Geometry check sheet. Reference: the model listing, model coordinates, mm. A direction names the side the tool comes from. Round coordinates to 2 decimals unless told otherwise and drop trailing zeros. Write each loop counter-clockwise with the first axis right and the second up, starting at its lowest first coordinate (ties: lowest second). Pieces come first, ordered by that corner, then holes.
Item 1: Cross-section at C-C (y = 29). Enter the section's corners in (x, z).
Item 2: Depth check by flat-ended pin: P1, Ø8, axis at x = 99, z = 47.5, coming from the +Y side; P2, Ø3, axis at x = 0.5, y = 48.5, coming from the +Z side; P3, Ø1.2, axis at x = 0.5, z = 57, coming from the +Y side. Enter the tip coordinate at first touch or a pass-through.
Item 3: Cross-section at A-A (x = -17.5). Enter the section's corners in (y, z), then the cut area to 3 significant figures.
Item 4: Access from +Z, -Z, +X, -X, +Y, -Y to the whole of each face (thin tool, end or side, straight path). Record for faces 1 (the face through (-83.213, 5.43, 32.045)), 2 (the face through (-98, 25, 32)), 3 (the face through (1, -25, 60)), 4 (the face through (-83.255, 14.7, 32.045)).
Item 5: Cross-section at B-B (z = 5). Enter the section's corners in (x, y), then the cut area to 3 significant figures.
Item 6: Cross-section at D-D (x = -95.5). Enter the section's corners in (y, z).
Item 7: Scan lines: probe 1 along X at (y, z) = (41.5, -7); probe 2 along X at (y, z) = (-26.5, 6); probe 3 along Z at (x, y) = (92, -11). Record each from-to range of solid material in increasing order.
Item 8: Draft check along X on faces 5 (the face through (105, 10, 0)), 6 (the face through (-106.262, -2.175, 32.045)), 7 (the face through (85.16, 0.425, 44.385)). Enter one of: pulls with the +X half, pulls with the -X half, needs draft (parallel to the pull), parting line crosses it, or undercut.
from build123d import *

# Parameters (mm, degrees)
BOSS_EXTRUDE1_DEPTH = 100
BOSS_EXTRUDE3_DEPTH = 65
SKETCH5_W           = 2.5
SKETCH5_H           = 50
CUT_EXTRUDE1_DEPTH  = 10
SKETCH6_W           = 2.5
SKETCH6_H           = 90
CUT_EXTRUDE3_DEPTH  = 5
SKETCH7_W           = 2.5
SKETCH7_H           = 70
CUT_EXTRUDE4_DEPTH  = 10
SKETCH8_W           = 2.5
SKETCH8_H           = 17.5
CUT_EXTRUDE5_DEPTH  = 5


with BuildPart() as part:
    # Sketch1 → Boss-Extrude1 (new body, symmetric)
    with BuildSketch(Plane(origin=(0, 0, 0), x_dir=(0, 0, -1), z_dir=(1, 0, 0))):
        Polygon((0, 0), (-55, 0), (-60, -5), (-60, -45), (-55, -50), (35, -50), (40, -45), (40, 45), (35, 50), (5, 50), (0, 45), align=None)
    extrude(amount=BOSS_EXTRUDE1_DEPTH, both=True)

    # Sketch2 → Boss-Extrude3 (add)
    with BuildSketch(Plane.XY):
        Polygon((113.271933364, 10), (110.259762125, 19.270509831), (102.373795443, 25), (92.626204557, 25), (84.740237875, 19.270509831), (81.728066636, 10), (84.740237875, 0.729490169), (92.626204557, -5), (102.373795443, -5), (110.259762125, 0.729490169), align=None)
    boss_extrude3 = extrude(amount=BOSS_EXTRUDE3_DEPTH)

    # Mirror1: Boss-Extrude3 across plane
    add(boss_extrude3.mirror(Plane(origin=(0, 0, 0), x_dir=(0, 0, 1), z_dir=(1, 0, 0))))

    # Sketch5 → Cut-Extrude1 (cut)
    with BuildSketch(Plane.XY):
        with Locations((0, 25)):
            Rectangle(SKETCH5_W, SKETCH5_H)
    extrude(amount=-CUT_EXTRUDE1_DEPTH, mode=Mode.SUBTRACT)

    # Sketch6 → Cut-Extrude3 (cut)
    with BuildSketch(Plane(origin=(0, 50, 0), x_dir=(1, 0, 0), z_dir=(0, 1, 0))):
        with Locations((0, -15)):
            Rectangle(SKETCH6_W, SKETCH6_H)
    extrude(amount=-CUT_EXTRUDE3_DEPTH, mode=Mode.SUBTRACT)

    # Sketch7 → Cut-Extrude4 (cut)
    with BuildSketch(Plane(origin=(0, 0, 0), x_dir=(1, 0, 0), z_dir=(0, 1, 0))):
        with Locations((0, -25)):
            Rectangle(SKETCH7_W, SKETCH7_H)
    extrude(amount=-CUT_EXTRUDE4_DEPTH, mode=Mode.SUBTRACT)

    # Sketch8 → Cut-Extrude5 (cut)
    with BuildSketch(Plane.XY.offset(60)):
        with Locations((0, -8.75)):
            Rectangle(SKETCH8_W, SKETCH8_H)
    extrude(amount=-CUT_EXTRUDE5_DEPTH, mode=Mode.SUBTRACT)


solid = part.part
Resolved:
1. outline: (-100, -40) - (100, -40) - (100, 0) - (1.25, 0) - (1.25, -10) - (-1.25, -10) - (-1.25, 0) - (-100, 0) - close
2. P1: stops at y = 25
2. P2: stops at z = -2.2
2. P3: stops at y = -17.5
3. outline: (-50, -35) - (-45, -40) - (45, -40) - (50, -35) - (50, -5) - (45, 0) - (0, 0) - (0, 55) - (-5, 60) - (-45, 60) - (-50, 55) - close
3. area: 6,940 mm2
4. face 1: +Z
4. face 2: +Z, +X, -X, +Y
4. face 3: +Z, +X, -X, -Y
4. face 4: +Z, +Y
5. outline: (-113.27, 10) - (-110.26, 0.73) - (-102.37, -5) - (-100, -5) - (-100, -50) - (100, -50) - (100, -5) - (102.37, -5) - (110.26, 0.73) - (113.27, 10) - (110.26, 19.27) - (102.37, 25) - (92.63, 25) - (84.74, 19.27) - (81.73, 10) - (84.74, 0.73) - (85.74, 0) - (1.25, 0) - (1.25, -10) - (-1.25, -10) - (-1.25, 0) - (-85.74, 0) - (-84.74, 0.73) - (-81.73, 10) - (-84.74, 19.27) - (-92.63, 25) - (-102.37, 25) - (-110.26, 19.27) - close
5. area: 11,300 mm2
6. outline: (-50, -35) - (-45, -40) - (45, -40) - (50, -35) - (50, -5) - (45, 0) - (25, 0) - (25, 65) - (-5, 65) - (-5, 60) - (-45, 60) - (-50, 55) - close
7. probe 1: x = -100 to -1.25, 1.25 to 100
7. probe 2: x = -100 to 100
7. probe 3: z = -40 to 60
8. face 5: needs draft
8. face 6: pulls with the -X half
8. face 7: undercut
